```python
from build123d import *

# Parameters (mm, degrees)
SKETCH_R    = 14.75
SKETCH001_R = 11
SKETCH002_W = 11
SKETCH002_H = 8
PAD_DEPTH   = 14
FILLET_R    = 4


with BuildPart() as part:
    # Sketch → AdditiveLoft section 0
    with BuildSketch(Plane.XY):
        Circle(SKETCH_R)
    # Sketch001 (on DatumPlane) → AdditiveLoft section 1
    with BuildSketch(Plane.XY.offset(20)):
        Circle(SKETCH001_R)
    loft()

    # Sketch002 (on Face1 of AdditiveLoft) → Pad (new body)
    with BuildSketch(Plane(origin=(0, 0, 0), x_dir=(1, 0, 0), z_dir=(0, 0, -1))):
        Rectangle(SKETCH002_W, SKETCH002_H)
    extrude(amount=PAD_DEPTH)

    # Fillet
    fillet_edges = [part.edges().sort_by_distance(p)[0] for p in [
        (5.5, 0, 0),
        (0, -4, 0),
        (0, 4, 0),
        (-5.5, 0, 0),
    ]]
    fillet(fillet_edges, radius=FILLET_R)


solid = part.part
```
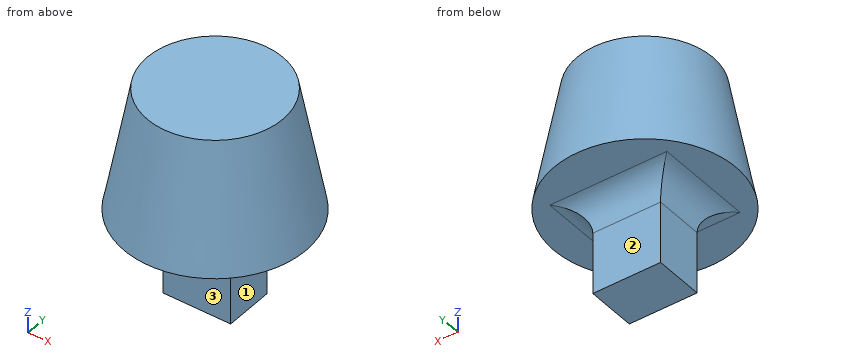
Verification items for the finished model (mm, model axes). Face numbers are marked on the shaded views. A direction names the side the tool comes from. Coordinates: 2 decimals unless noted, no trailing zeros. Write each loop counter-clockwise with the first axis right and the second up, starting at its lowest first coordinate (ties: lowest second). Pieces come first, ordered by that corner, then holes. Notation, with made-up numbers: (62, -26.5) - (76, -26.5) arc R17 ccw to (76, -15.5) - close; hole circle Ø4 at (73, -8). An arc over 180 degrees is marked (long way). One line per question, with ' | ' between items. Start each with the question number.
1. Section check C-C (z = -8). Enter the section's corners in (x, y), plus the area to 3 significant figures.
2. Section check B-B (z = 8). Enter the section's corners in (x, y), plus the area to 3 significant figures.
3. Section check A-A (x = 0). Enter the section's corners in (y, z), plus the area to 3 significant figures.
4. Access from +Z, -Z, +X, -X, +Y, -Y to the whole of each face (thin tool, end or side, straight path). Record for the marked faces 1, 2 and 3.
5. Section check D-D (z = -3). Enter the section's corners in (x, y), plus the area to 3 significant figures.
6. Gauge pin test, flat ends, axial feed: P1, Ø4, axis at y = -7.5, z = 8, coming from the +X side; P2, Ø8, axis at x = 1.5, z = -10, coming from the +Y side; P3, Ø1, axis at x = 1, z = -1, coming from the +Y side. Record the tip position at first contact, or that the pin passes through.
7. Material ranges on line 1 along X through (y, z) = (-1.75, -6); line 2 along Y through (x, z) = (0, 15.5); line 3 along Y through (x, z) = (-1, 14.5), recorded low to high.
Computed values:
1) outline: (-5.5, -4) - (5.5, -4) - (5.5, 4) - (-5.5, 4) - close | area: 88.0 mm²
2) outline: circle Ø26.5 at (0, 0) | area: 552 mm²
3) outline: (-14.75, 0) - (-8, 0) arc R4 cw to (-4, -4) - (-4, -14) - (4, -14) - (4, -4) arc R4 cw to (8, 0) - (14.75, 0) - (11, 20) - (-11, 20) - close | area: 634 mm²
4) face 1: -Z, +X, +Y, -Y | face 2: -Z, +X, -X, +Y | face 3: -Z, +X, -X, -Y
5) outline: (-5.63, -4.13) - (5.63, -4.13) - (5.63, 4.13) - (-5.63, 4.13) - close | area: 92.9 mm²
6) P1: x = 12.14 | P2: y = 4 | P3: y = 6.06
7) line 1: -5.5 to 5.5 | line 2: -11.84 to 11.84 | line 3: -11.99 to 11.99
